Read the model definition and answer for the solid it produces. Units are mm, in the model's axes. Coordinates: 2 decimals unless noted, no trailing zeros. Write each loop counter-clockwise with the first axis right and the second up, starting at its lowest first coordinate (ties: lowest second). Pieces come first, ordered by that corner, then holes.
from build123d import *

# Parameters (mm, degrees)
F0_R     = 48.167809
F1_DEPTH = 10
F2_R     = 38.085583
F3_DEPTH = 5
F5_DEPTH = 3
F6_R     = 1


with BuildPart() as f1:
    # F0 (on Top) → F1 (new body)
    with BuildSketch(Plane.XY):
        with Locations((38.1, -38.1)):
            Circle(F0_R)
    extrude(amount=F1_DEPTH)

    # F2 (on face) → F3 (join)
    with BuildSketch(Plane.XY.offset(10)):
        with Locations((38.1, -38.1)):
            Circle(F2_R)
    extrude(amount=F3_DEPTH)

    # F4 (on face) → F5 (cut)
    with BuildSketch(Plane.XY.offset(15)):
        Polygon((22.775168, -31.485546), (18.479863, -31.485546), (18.522732, -44.620931), (21.934504, -44.620931), (21.934504, -36.083298), (27.067889, -44.620931), (30.365812, -44.620931), (30.365812, -31.485546), (27.093198, -31.485546), (27.093198, -38.667116), align=None)
        with BuildLine():
            Line((37.025582, -31.485546), (33.525705, -31.485546))
            Line((33.525705, -31.485546), (33.525705, -39.915241))
            ThreePointArc((33.525705, -39.915241), (39.355047, -44.941114), (45.184389, -39.915241))
            Line((45.184389, -39.915241), (45.184389, -31.485546))
            Line((45.184389, -31.485546), (41.616332, -31.485546))
            Line((41.616332, -31.485546), (41.616332, -39.915241))
            ThreePointArc((41.616332, -39.915241), (39.320957, -42.210616), (37.025582, -39.915241))
            Line((37.025582, -39.915241), (37.025582, -31.485546))
        make_face()
        Polygon((58.469679, -31.485546), (46.738543, -31.485546), (46.738543, -34.295145), (50.627492, -34.295145), (50.627492, -44.531766), (54.387886, -44.531766), (54.387886, -34.295145), (58.469679, -34.295145), align=None)
    extrude(amount=-F5_DEPTH, mode=Mode.SUBTRACT)

    # F6
    f6_edges = [f1.edges().sort_by_distance(p)[0] for p in [
        (-10.067809, -38.1, 10),
        (0.014417, -38.1, 15),
    ]]
    fillet(f6_edges, radius=F6_R)


solid = f1.part
Item 1: The part is cut by section A-A (z = 1.75). Give the vertices of the cut face in (x, y).
Item 2: Given pin 1 (2 mm diameter, centred on y = -18, z = 8.5, fed in from -X); pin 2 (0.9 mm diameter, centred on x = 35, z = 14, fed in from -Y); pin 3 (0.9 mm diameter, centred on y = -36.5, z = 13, fed in from -X), each flat-ended and moving along its own axis, determine where each tip first touches the part or whether it passes through.
Item 3: Find the intervals of material crossed by probe 1 along Z at (x, y) = (29, -36.5); probe 2 along Z at (x, y) = (-1, -34); probe 3 along Y at (x, z) = (39, 5.5), in increasing order.
Item 4: Determine the mould class of faces 1 (the cylindrical face through (82.595, -56.549, 4.437)), 2 (the flat face through (29, -31.486, 14)), 3 (the flat face through (38, -38, 15)) for opening direction Y: +Y half, -Y half, draft (parallel to the pull), parting line (faces both ways), or undercut.
Answer:
1. outline: circle Ø96.34 at (38.1, -38.1)
2. pin 1: stops at x = -6.12
2. pin 2: stops at y = -76.09
2. pin 3: stops at x = 0.03
3. probe 1: z = 0 to 12
3. probe 2: z = 0 to 10
3. probe 3: y = -86.26 to 10.06
4. face 1: parting line
4. face 2: undercut
4. face 3: draft
